```python
from build123d import *

# Parameters (mm, degrees)
SKETCH1_W               = 16
SKETCH1_H               = 16
BOSS_EXTRUDE1_DEPTH     = 24
SKETCH12_W              = 12.4
SKETCH12_H              = 12.4
CUT_EXTRUDE6_DEPTH      = 22
SKETCH13_R              = 20
BOSS_EXTRUDE2_DEPTH     = 3
CHAMFER1_SIZE           = 2.5
SKETCH14_W              = 16
SKETCH14_H              = 16
BOSS_EXTRUDE3_DEPTH     = 12
CUT_EXTRUDE1_DEPTH      = 7.5
CUT_EXTRUDE5_DEPTH      = 6.3
CUT_EXTRUDE5_DEPTH_BACK = 0.1
SKETCH11_W              = 4.2
SKETCH11_H              = 5.5
CHAMFER2_SIZE           = 2
CHAMFER4_SIZE           = 2
SKETCH15_R              = 1.3
CUT_EXTRUDE7_DEPTH      = 42.620307543
CHAMFER5_SIZE           = 1
ESQUISSE3_W             = 15.926523834
ESQUISSE3_H             = 12
BOSS_EXTRU_1_DEPTH      = 5
ENL_V_MAT_EXTRU_1_DEPTH = 7
ESQUISSE5_R             = 1.3
ENL_V_MAT_EXTRU_2_DEPTH = 5
CHANFREIN2_SIZE         = 2
CHANFREIN3_SIZE         = 2
CHANFREIN4_SIZE         = 2


with BuildPart() as part:
    # Sketch1 → Boss-Extrude1 (new body)
    with BuildSketch(Plane(origin=(0, 0, 0), x_dir=(1, 0, 0), z_dir=(0, 1, 0))):
        with Locations((0, 8)):
            Rectangle(SKETCH1_W, SKETCH1_H)
    extrude(amount=BOSS_EXTRUDE1_DEPTH)

    # Sketch12 → Cut-Extrude6 (cut)
    with BuildSketch(Plane(origin=(0, 24, 0), x_dir=(1, 0, 0), z_dir=(0, 1, 0))):
        with Locations((0, 8)):
            Rectangle(SKETCH12_W, SKETCH12_H)
    extrude(amount=-CUT_EXTRUDE6_DEPTH, mode=Mode.SUBTRACT)

    # Sketch13 → Boss-Extrude2 (add)
    with BuildSketch(Plane(origin=(0, 0, 0), x_dir=(1, 0, 0), z_dir=(0, 1, 0))):
        with Locations(Location((0, 8, 0), (0, 0, 270))):
            Circle(SKETCH13_R)
    extrude(amount=BOSS_EXTRUDE2_DEPTH)

    # Chamfer1
    chamfer1_edges = [part.edges().sort_by_distance(p)[0] for p in [
        (0, 3, -28),
    ]]
    chamfer(chamfer1_edges, length=CHAMFER1_SIZE)

    # Sketch14 → Boss-Extrude3 (add)
    with BuildSketch(Plane(origin=(0, 3, 0), x_dir=(1, 0, 0), z_dir=(0, 1, 0))):
        Polygon((-8, 23), (8, 23), (9, 23), (9, -4), (8, -4), (-8, -4), (-9, -4), (-9, 23), align=None)
        with Locations((0, 8)):
            Rectangle(SKETCH14_W, SKETCH14_H, mode=Mode.SUBTRACT)
    extrude(amount=BOSS_EXTRUDE3_DEPTH)

    # Sketch5 → Cut-Extrude1 (cut)
    with BuildSketch(Plane(origin=(0, 0, -23), x_dir=(-1, 0, 0), z_dir=(0, 0, -1))):
        with BuildLine():
            Line((-2.1, 11.1), (2.1, 11.1))
            Line((2.1, 11.1), (3.1, 10.1))
            Line((3.1, 10.1), (3.1, 8.8))
            ThreePointArc((3.1, 8.8), (3.9, 8), (3.1, 7.2))
            Line((3.1, 7.2), (3.1, 4.9))
            Line((3.1, 4.9), (-3.1, 4.9))
            Line((-3.1, 4.9), (-3.1, 7.2))
            ThreePointArc((-3.1, 7.2), (-3.9, 8), (-3.1, 8.8))
            Line((-3.1, 8.8), (-3.1, 10.1))
            Line((-3.1, 10.1), (-2.1, 11.1))
        make_face()
    extrude(amount=-CUT_EXTRUDE1_DEPTH, mode=Mode.SUBTRACT)

    # Sketch11 → Cut-Extrude5 (cut, two sides: drawn at the far end of the back side and taken through both)
    with BuildSketch(Plane.XZ.offset(-11.1).offset(-CUT_EXTRUDE5_DEPTH_BACK)):
        with Locations((0, -18.25)):
            Rectangle(SKETCH11_W, SKETCH11_H)
    extrude(amount=CUT_EXTRUDE5_DEPTH + CUT_EXTRUDE5_DEPTH_BACK, mode=Mode.SUBTRACT)

    # Chamfer2
    chamfer2_edges = [part.edges().sort_by_distance(p)[0] for p in [
        (0, 15, -23),
        (9, 9, -23),
        (-9, 9, -23),
    ]]
    chamfer(chamfer2_edges, length=CHAMFER2_SIZE)

    # Chamfer4
    chamfer4_edges = [part.edges().sort_by_distance(p)[0] for p in [
        (0, 15, 4),
        (-9, 9, 4),
        (9, 9, 4),
    ]]
    chamfer(chamfer4_edges, length=CHAMFER4_SIZE)

    # Sketch15 → Cut-Extrude7 (cut, through all)
    with BuildSketch(Plane(origin=(0, 0, -15.5), x_dir=(-1, 0, 0), z_dir=(0, 0, -1))):
        with Locations((0, 8)):
            Circle(SKETCH15_R)
    extrude(amount=-CUT_EXTRUDE7_DEPTH, mode=Mode.SUBTRACT)

    # Chamfer5
    chamfer5_edges = [part.edges().sort_by_distance(p)[0] for p in [
        (0, 24, -16),
        (-8, 24, -8),
        (0, 24, 0),
        (8, 24, -8),
    ]]
    chamfer(chamfer5_edges, length=CHAMFER5_SIZE)

    # Esquisse3 → Boss.-Extru.1 (add)
    with BuildSketch(Plane.ZY.offset(9)):
        with Locations((-7.963261917, 9)):
            Rectangle(ESQUISSE3_W, ESQUISSE3_H)
    extrude(amount=BOSS_EXTRU_1_DEPTH)

    # Esquisse4 → Enlèv. mat.-Extru.1 (cut)
    with BuildSketch(Plane.ZY.offset(14)):
        with BuildLine():
            Line((-10.065, 11.1), (-5.865, 11.1))
            Line((-5.865, 11.1), (-4.865, 10.1))
            Line((-4.865, 10.1), (-4.865, 8.8))
            ThreePointArc((-4.865, 8.8), (-4.065, 8), (-4.865, 7.2))
            Line((-4.865, 7.2), (-4.865, 4.9))
            Line((-4.865, 4.9), (-11.065, 4.9))
            Line((-11.065, 4.9), (-11.065, 7.2))
            ThreePointArc((-11.065, 7.2), (-11.865, 8), (-11.065, 8.8))
            Line((-11.065, 8.8), (-11.065, 10.1))
            Line((-11.065, 10.1), (-10.065, 11.1))
        make_face()
    extrude(amount=-ENL_V_MAT_EXTRU_1_DEPTH, mode=Mode.SUBTRACT)

    # Esquisse5 → Enlèv. mat.-Extru.2 (cut)
    with BuildSketch(Plane.ZY.offset(7)):
        with Locations((-7.965, 8)):
            Circle(ESQUISSE5_R)
    extrude(amount=-ENL_V_MAT_EXTRU_2_DEPTH, mode=Mode.SUBTRACT)

    # Chanfrein2
    chanfrein2_edges = [part.edges().sort_by_distance(p)[0] for p in [
        (-14, 15, -7.963261917),
    ]]
    chamfer(chanfrein2_edges, length=CHANFREIN2_SIZE)

    # Chanfrein3
    chanfrein3_edges = [part.edges().sort_by_distance(p)[0] for p in [
        (-14, 8, 0),
    ]]
    chamfer(chanfrein3_edges, length=CHANFREIN3_SIZE)

    # Chanfrein4
    chanfrein4_edges = [part.edges().sort_by_distance(p)[0] for p in [
        (-14, 8, -15.926523834),
    ]]
    chamfer(chanfrein4_edges, length=CHANFREIN4_SIZE)


solid = part.part
```
Source: CAD feature listing. Evaluate the final solid. Frame: model axes, mm. A direction names the side the tool comes from. Coordinates: 2 decimals unless noted, no trailing zeros. Write each loop counter-clockwise with the first axis right and the second up, starting at its lowest first coordinate (ties: lowest second). Pieces come first, ordered by that corner, then holes. Notation, with made-up numbers: (12, 42.25) - (44, 42.25) arc R21 ccw to (44, 69.25) - close; hole circle Ø7 at (-28.5, 14). An arc over 180 degrees is marked (long way). Answer as a JSON object with one key per item and string values.
Q1. First-contact query: pin 1 Ø2.5 at (x, y) = (-10, 8.5) entering from -Z; pin 2 Ø1 at (x, z) = (14.5, 4) entering from -Y; pin 3 Ø6 at (x, y) = (-2, 8.5) entering from +Z; pin 4 Ø2 at (x, z) = (-4, 2.5) entering from +Y. Flat tips, straight axial feed; report the tip coordinate or a pass-through.
Ans:
{"pin 1": "stops at z = -21.25", "pin 2": "stops at y = 0", "pin 3": "stops at z = 4", "pin 4": "stops at y = 15"}
Q2. Draft query along Y for faces 6 (the flat face through (9, 9, -10)), 7 (the flat face through (-7.5, 23.5, -7.9)), 8 (the flat face through (-3.1, 6, -19)). Return one class per face: released by +Y, released by -Y, zero draft, split by the parting line, or undercut.
Ans:
{"face 6": "zero draft", "face 7": "released by +Y", "face 8": "undercut"}
Q3. Section query C-C, the plane x = 0. State how many separate pieces and enclosed holes the cut face has, plus the area to 3 significant figures.
Ans:
{"separate pieces": "3", "enclosed holes": "0", "area": "250 mm2"}
Q4. Section query A-A, the plane y = 21. Output: boundary loops of the cut face in (x, z), plus the area to 3 significant figures.
Ans:
{"outline": "(-8, -16) - (8, -16) - (8, 0) - (-8, 0) - close; hole (-6.2, -14.2) - (6.2, -14.2) - (6.2, -1.8) - (-6.2, -1.8) - close", "area": "102 mm2"}
Q5. Set-up query: faces 1 (the flat face through (-11, 6, -11.065)), 2 (the flat face through (0.1, 11.3, -23)), 3 (the flat face through (-9, 9, 1)), 4 (the flat face through (0, 14, -14.2)), 5 (the cylindrical face through (3.9, 8, -19.3)). Return all of +Z, -Z, +X, -X, +Y, -Y with unobstructed straight access to the full face (end or side cutting, diameter ignored); none if empty.
Ans:
{"face 1": "-X", "face 2": "-Z, +X, -X, +Y", "face 3": "+Z, -X, +Y", "face 4": "+Y", "face 5": "-Z"}
Q6. Material intervals for line 1 (Y direction, x = 0, z = -14.85); line 2 (Z direction, x = 5.5, y = 6); line 3 (X direction, y = 22.75, z = -2.5), sorted ascending. Write a range as [from, to].
Ans:
{"line 1": "y = [0, 6.7], [9.3, 24]", "line 2": "z = [-23, -14.2], [-1.8, 4]", "line 3": "x = [-8, -6.2], [6.2, 8]"}
